For this review, take the finished solid that the model builds, in its own axes (mm). Round coordinates to 2 decimals unless told otherwise and drop trailing zeros. Order: outer loops, then holes, each group sorted by start corner. A loop starts at its lowest first (then second) coordinate and runs counter-clockwise, first axis right, second up.
from build123d import *

# Parameters (mm, degrees)
BASEFLANGE_W                   = 50
BASEFLANGE_H                   = 2050
BASE_FLANGE1_DEPTH             = 2
EDGE_FLANGE1_STRIP_W           = 10
EDGE_FLANGE1_STRIP_H           = 2
EDGE_FLANGE1_STRIP_CUT_DEPTH   = 2050
EDGE_FLANGE1_STRIP_2_W         = 10
EDGE_FLANGE1_STRIP_2_H         = 2
EDGE_FLANGE1_STRIP_CUT_2_DEPTH = 2050
EDGE_FLANGE1_DEPTH             = 2050
EDGE_FLANGE1_BEND_DEPTH        = 2050
EDGE_FLANGE2_STRIP_W           = 10
EDGE_FLANGE2_STRIP_H           = 2
EDGE_FLANGE2_STRIP_CUT_DEPTH   = 2050
EDGE_FLANGE2_STRIP_2_W         = 10
EDGE_FLANGE2_STRIP_2_H         = 2
EDGE_FLANGE2_STRIP_CUT_2_DEPTH = 2050
EDGE_FLANGE2_DEPTH             = 2050
EDGE_FLANGE2_BEND_DEPTH        = 2050
SKETCH18_R                     = 1.6
CUT_EXTRUDE1_DEPTH             = 1026.609574838


# Sheet-metal steps are written as plain solids
with BuildPart() as part:
    # BaseFlange → Base-Flange1 (new body)
    with BuildSketch(Plane.XY):
        Rectangle(BASEFLANGE_W, BASEFLANGE_H)
    extrude(amount=BASE_FLANGE1_DEPTH)

    # Edge-Flange1 strip (across the edge) → Edge-Flange1 strip cut (cut)
    with BuildSketch(Plane(origin=(25, -1025, 2), x_dir=(-1, 0, 0), z_dir=(0, 1, 0))):
        with Locations((-2, -1)):
            Rectangle(EDGE_FLANGE1_STRIP_W, EDGE_FLANGE1_STRIP_H)
    extrude(amount=EDGE_FLANGE1_STRIP_CUT_DEPTH, mode=Mode.SUBTRACT)

    # Edge-Flange1 strip 2 (across the edge) → Edge-Flange1 strip cut 2 (cut)
    with BuildSketch(Plane(origin=(-25, 1025, 2), x_dir=(1, 0, 0), z_dir=(0, -1, 0))):
        with Locations((-2, -1)):
            Rectangle(EDGE_FLANGE1_STRIP_2_W, EDGE_FLANGE1_STRIP_2_H)
    extrude(amount=EDGE_FLANGE1_STRIP_CUT_2_DEPTH, mode=Mode.SUBTRACT)

    # Edge-Flange1 section (across the edge) → Edge-Flange1 (add)
    with BuildSketch(Plane(origin=(25, -1025, 2), x_dir=(-1, 0, 0), z_dir=(0, 1, 0))):
        with BuildLine():
            Line((0, 1), (0, 23))
            Line((0, 23), (2, 23))
            Line((2, 23), (2, 1))
            ThreePointArc((2, 1), (2.292893219, 0.292893219), (3, 0))
            Line((3, 0), (3, -2))
            ThreePointArc((3, -2), (0.878679656, -1.121320344), (0, 1))
        make_face()
    extrude(amount=EDGE_FLANGE1_DEPTH)

    # Edge-Flange1 section 2 (across the edge) → Edge-Flange1 bend (add)
    with BuildSketch(Plane(origin=(-25, 1025, 2), x_dir=(1, 0, 0), z_dir=(0, -1, 0))):
        with BuildLine():
            Line((0, 1), (0, 23))
            Line((0, 23), (2, 23))
            Line((2, 23), (2, 1))
            ThreePointArc((2, 1), (2.292893219, 0.292893219), (3, 0))
            Line((3, 0), (3, -2))
            ThreePointArc((3, -2), (0.878679656, -1.121320344), (0, 1))
        make_face()
    extrude(amount=EDGE_FLANGE1_BEND_DEPTH)

    # Edge-Flange2 strip (across the edge) → Edge-Flange2 strip cut (cut)
    with BuildSketch(Plane(origin=(-23, 1025, 25), x_dir=(0, 0, -1), z_dir=(0, -1, 0))):
        with Locations((-2, -1)):
            Rectangle(EDGE_FLANGE2_STRIP_W, EDGE_FLANGE2_STRIP_H)
    extrude(amount=EDGE_FLANGE2_STRIP_CUT_DEPTH, mode=Mode.SUBTRACT)

    # Edge-Flange2 strip 2 (across the edge) → Edge-Flange2 strip cut 2 (cut)
    with BuildSketch(Plane(origin=(23, -1025, 25), x_dir=(0, 0, -1), z_dir=(0, 1, 0))):
        with Locations((-2, -1)):
            Rectangle(EDGE_FLANGE2_STRIP_2_W, EDGE_FLANGE2_STRIP_2_H)
    extrude(amount=EDGE_FLANGE2_STRIP_CUT_2_DEPTH, mode=Mode.SUBTRACT)

    # Edge-Flange2 section (across the edge) → Edge-Flange2 (add)
    with BuildSketch(Plane(origin=(-23, 1025, 25), x_dir=(0, 0, -1), z_dir=(0, -1, 0))):
        with BuildLine():
            Line((0, 1), (0, 8))
            Line((0, 8), (2, 8))
            Line((2, 8), (2, 1))
            ThreePointArc((2, 1), (2.292893219, 0.292893219), (3, 0))
            Line((3, 0), (3, -2))
            ThreePointArc((3, -2), (0.878679656, -1.121320344), (0, 1))
        make_face()
    extrude(amount=EDGE_FLANGE2_DEPTH)

    # Edge-Flange2 section 2 (across the edge) → Edge-Flange2 bend (add)
    with BuildSketch(Plane(origin=(23, -1025, 25), x_dir=(0, 0, -1), z_dir=(0, 1, 0))):
        with BuildLine():
            Line((0, 1), (0, 8))
            Line((0, 8), (2, 8))
            Line((2, 8), (2, 1))
            ThreePointArc((2, 1), (2.292893219, 0.292893219), (3, 0))
            Line((3, 0), (3, -2))
            ThreePointArc((3, -2), (0.878679656, -1.121320344), (0, 1))
        make_face()
    extrude(amount=EDGE_FLANGE2_BEND_DEPTH)

    # Sketch18 → Cut-Extrude1 (cut, through all)
    with BuildSketch(Plane.XY):
        with Locations(Location((0, -17.5, 0), (0, 0, 180))):
            Circle(SKETCH18_R)
        with Locations(Location((0, -942.5, 0), (0, 0, 180))):
            Circle(SKETCH18_R)
        with Locations(Location((0, 942.5, 0), (0, 0, 180))):
            Circle(SKETCH18_R)
        with Locations(Location((0, -907.5, 0), (0, 0, 180))):
            Circle(SKETCH18_R)
        with Locations(Location((0, 17.5, 0), (0, 0, 180))):
            Circle(SKETCH18_R)
        with Locations(Location((0, 907.5, 0), (0, 0, 180))):
            Circle(SKETCH18_R)
    extrude(amount=CUT_EXTRUDE1_DEPTH, mode=Mode.SUBTRACT)


solid = part.part
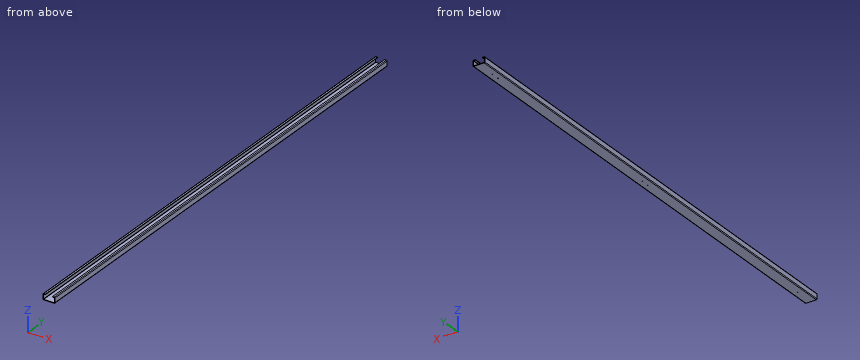
(1) Wall thickness on L1, parallel to X at y = -718, z = 10.5; L2, parallel to Z at x = -4, y = -680.5; L3, parallel to Z at x = -20, y = 522.5: over which ranges is each line inside the solid? List them lowest first.
(2) Add section A-A on z = 9. Give the boundary of the cut face in (x, y).
(3) Add section B-B on y = -844.5. Give the boundary of the cut face in (x, z).
(4) Clearance check with flat-ended pins moving along their axes: P1, Ø1.6, axis at y = 35.5, z = 24, coming from the +X side; P2, Ø12, axis at x = 19.5, z = 7.5, coming from the -Y side; P3, Ø2.5, axis at x = 0, y = -942.5, coming from the +Z side; P4, Ø4, axis at x = 3.5, y = 162.5, coming from the +Z side. State where each tip first meets the part, or that it passes through.
Here are the results:
1. L1: x = -25 to -23, 23 to 25
1. L2: z = 0 to 2
1. L3: z = 0 to 2, 23 to 25
2. outline: (-25, -1025) - (-23, -1025) - (-23, 1025) - (-25, 1025) - close; (23, -1025) - (25, -1025) - (25, 1025) - (23, 1025) - close
3. outline: (-25, 3) arc R3 ccw to (-22, 0) - (22, 0) arc R3 ccw to (25, 3) - (25, 22) arc R3 ccw to (22, 25) - (15, 25) - (15, 23) - (22, 23) arc R1 cw to (23, 22) - (23, 3) arc R1 cw to (22, 2) - (-22, 2) arc R1 cw to (-23, 3) - (-23, 22) arc R1 cw to (-22, 23) - (-15, 23) - (-15, 25) - (-22, 25) arc R3 ccw to (-25, 22) - close
4. P1: stops at x = 24.75
4. P2: stops at y = -1025
4. P3: passes through
4. P4: stops at z = 2
